Geometry check sheet. Reference: drawing and pictorial views, mm from the part's lowest x, y, z. A direction names the side the tool comes from. Give positions to 0.01 mm unless a question says otherwise; leave off trailing zeros. Loops run counter-clockwise (first coordinate to the right, second up) from the corner with the lowest first, then second, coordinate; pieces in that order, holes last. Notation, with made-up numbers: (-4.5, 61) -> (2.5, 61) arc R10 ccw to (2.5, 73) -> close; hole circle Ø7 at (86, 85.5). An arc over 180 degrees is marked (long way). Write item = value, one per line. Start each with the question number.
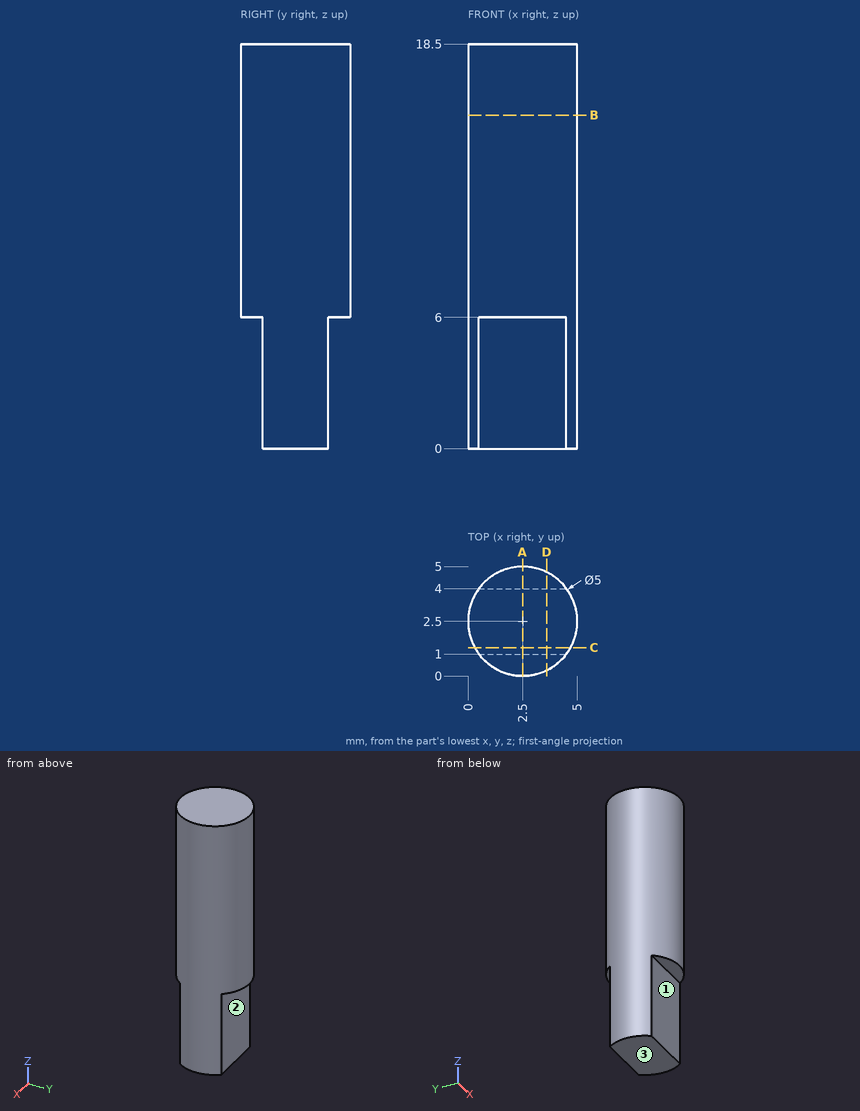
1) Section check A-A (x = 2.5). Enter the section's corners in (y, z), plus the area to 3 significant figures.
2) Thickness scan on line 1 (Z direction, x = 3.2, y = 0.9); line 2 (X direction, y = 2.65, z = 1.5); line 3 (Y direction, x = 2.2, z = 4). Record the ranges inside material, lowest first.
3) Section check B-B (z = 15.25). Enter the section's corners in (x, y), plus the area to 3 significant figures.
4) Depth check by flat-ended pin: pin 1 Ø1 at (x, z) = (1.5, 5) entering from -Y; pin 2 Ø1 at (x, z) = (0.5, 13.5) entering from +Y; pin 3 Ø0.5 at (x, y) = (2, 0.5) entering from -Z. Enter the tip coordinate at first touch or a pass-through.
5) Tool access check on the marked faces 1, 2 and 3. Record the directions out of +Z, -Z, +X, -X, +Y, -Y that give a thin tool (end or side, any length) a straight path to the whole face; none if there is none.
6) Section check C-C (y = 1.3). Enter the section's corners in (x, z), plus the area to 3 significant figures.
7) Section check D-D (x = 3.6). Enter the section's corners in (y, z) (3 decimals).
Check result:
q1.outline = (0, 6) -> (1, 6) -> (1, 0) -> (4, 0) -> (4, 6) -> (5, 6) -> (5, 18.5) -> (0, 18.5) -> close
q1.area = 80.5 mm2
q2.line_1 = 6 to 18.5
q2.line_2 = 0 to 5
q2.line_3 = 1 to 4
q3.outline = circle Ø5 at (2.5, 2.5)
q3.area = 19.6 mm2
q4.pin_1 = 1
q4.pin_2 = 4.5
q4.pin_3 = 6
q5.face_1 = -Z, +X, -X, -Y
q5.face_2 = -Z, +X, -X, +Y
q5.face_3 = -Z, +X, -X, +Y, -Y
q6.outline = (0.31, 0) -> (4.69, 0) -> (4.69, 18.5) -> (0.31, 18.5) -> close
q6.area = 81.1 mm2
q7.outline = (0.255, 6) -> (1, 6) -> (1, 0) -> (4, 0) -> (4, 6) -> (4.745, 6) -> (4.745, 18.5) -> (0.255, 18.5) -> close
